```python
from build123d import *

# Parameters (mm, degrees)
F0_R          = 12.5
F1_DEPTH      = 100
F2_R          = 9.5
F3_DEPTH      = 90
F3_DEPTH_BACK = 101.346
F4_R          = 11
F5_DEPTH      = 10
F5_DEPTH_BACK = 25.4


with BuildPart() as f1:
    # F0 (on Top) → F1 (new body)
    with BuildSketch(Plane.XY):
        Circle(F0_R)
    extrude(amount=F1_DEPTH)

    # F2 (on face) → F3 (cut, two sides)
    with BuildSketch(Plane(origin=(0, 0, 0), x_dir=(1, 0, 0), z_dir=(0, 0, -1))) as f3_sk:
        Circle(F2_R)
    extrude(amount=-F3_DEPTH, mode=Mode.SUBTRACT)
    extrude(f3_sk.sketch, amount=F3_DEPTH_BACK, mode=Mode.SUBTRACT)

    # F4 (on face) → F5 (cut, two sides)
    with BuildSketch(Plane.XY.offset(100)) as f5_sk:
        Circle(F4_R)
    extrude(amount=-F5_DEPTH, mode=Mode.SUBTRACT)
    extrude(f5_sk.sketch, amount=F5_DEPTH_BACK, mode=Mode.SUBTRACT)


solid = f1.part
```
For this review, take the finished solid that the model builds, in its own axes (mm). A direction names the side the tool comes from. Round coordinates to 2 decimals unless told otherwise and drop trailing zeros. Loops run counter-clockwise (first coordinate to the right, second up) from the corner with the lowest first, then second, coordinate; pieces in that order, holes last.
Q1. Mouldability with a two-part tool opening along X and no side actions: class faces 3 (the face through (11.923, 3.755, 49.3)), 4 (the face through (4.38, 8.43, 44.37)), 5 (the face through (5, -10, 100)) as +X half, -X half, draft (parallel to the pull), parting line (faces both ways), or undercut.
Result sheet:
face 3: parting line
face 4: undercut
face 5: draft
Q2. Add section C-C on z = 91. Write out the cut boundary in (x, y), plus the area to 3 significant figures.
Result sheet:
outline: circle Ø25 at (0, 0); hole circle Ø22 at (0, 0)
area: 111 mm2
Q3. Insertion check: pin 1 Ø8 at (y, z) = (8.5, 67) entering from +X; pin 2 Ø11 at (x, y) = (-3.5, -2.5) entering from +Z; pin 3 Ø5 at (x, z) = (9, 71) entering from -Y. Each pin has a flat end and moves straight along its axis. Give the tip position at first contact, or say it passes through.
Result sheet:
pin 1: stops at x = 11.66
pin 2: stops at z = 90
pin 3: stops at y = -10.68
Q4. Add section D-D on z = 79.5. Write out the cut boundary in (x, y).
Result sheet:
outline: circle Ø25 at (0, 0); hole circle Ø19 at (0, 0)
Q5. Add section A-A on x = 0. Write out the cut boundary in (y, z).
Result sheet:
outline: (-12.5, 0) - (-9.5, 0) - (-9.5, 90) - (-11, 90) - (-11, 100) - (-12.5, 100) - close; (9.5, 0) - (12.5, 0) - (12.5, 100) - (11, 100) - (11, 90) - (9.5, 90) - close
Q6. To check wall thickness, follow line 1 along Y through (x, z) = (0, 92.25); line 2 along Y through (x, z) = (0, 18); line 3 along Z through (x, y) = (6.75, -8). State the ranges of each line that lie inside material, in increasing order.
Result sheet:
line 1: y = -12.5 to -11, 11 to 12.5
line 2: y = -12.5 to -9.5, 9.5 to 12.5
line 3: z = 0 to 90
Q7. Machinability: for faces 1 (the face through (2.7, 9.3, 0)), 2 (the face through (-2.38, -10.74, 95.07)), which of the approach directions +Z, -Z, +X, -X, +Y, -Y give a long, thin tool a straight path to every point of the face, cutting with its end or side? Answer none if there is none.
Result sheet:
face 1: -Z, +X, -X, +Y, -Y
face 2: +Z
